The listing builds one solid part. Answer for the finished solid, in the listing's coordinates (mm). Coordinates: 2 decimals unless noted, no trailing zeros. Write each loop counter-clockwise with the first axis right and the second up, starting at its lowest first coordinate (ties: lowest second). Pieces come first, ordered by that corner, then holes. Notation, with made-up numbers: M 39.5,28.25 L 63.5,28.25 A13 cw 63.5,52.25 Z; hole C 46.25,17 d1. An arc over 180 degrees is marked long. Answer as a JSON object with one key per item and string values. Group by question number.
from build123d import *

# Parameters (mm, degrees)
F0_R     = 100
F0_R_2   = 20
F1_DEPTH = 12.5


with BuildPart() as f1:
    # F0 (on Top) → F1 (new body)
    with BuildSketch(Plane.XY):
        with BuildLine():
            ThreePointArc((205.158335, -0.516176), (96.574996, 55.7576), (102.132146, 177.930417))
            ThreePointArc((102.132146, 177.930417), (0, 375), (-102.132146, 177.930417))
            ThreePointArc((-102.132146, 177.930417), (-96.574996, 55.7576), (-205.158335, -0.516176))
            ThreePointArc((-205.158335, -0.516176), (-324.759526, -187.5), (-103.026189, -177.414242))
            ThreePointArc((-103.026189, -177.414242), (0, -111.5152), (103.026189, -177.414242))
            ThreePointArc((103.026189, -177.414242), (324.759526, -187.5), (205.158335, -0.516176))
        make_face()
        Circle(F0_R, mode=Mode.SUBTRACT)
        Circle(F0_R)
        Circle(F0_R_2, mode=Mode.SUBTRACT)
    extrude(amount=F1_DEPTH)


solid = f1.part
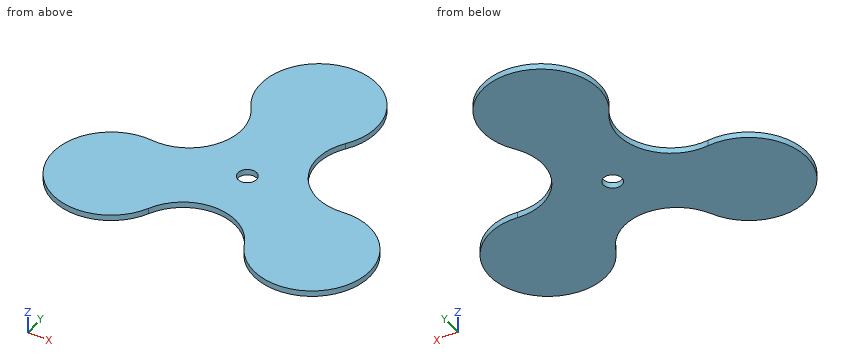
Item 1: A cutting plane is placed at A-A, the plane x = 0. Write down the section's boundary in (y, z).
Item 2: A cutting plane is placed at D-D, the plane x = -144. Write down the section's boundary in (y, z), and give its area (3 significant figures).
Item 3: A cutting plane is placed at C-C, the plane z = 8.5. Write down the section's boundary in (x, y).
Item 4: A flat-ended cylindrical pin translates along its axis: pin 1 Ø5 at (x, z) = (176, 11) entering from -Y. Find the tip coordinate at first contact, or state that the pin passes through.
Item 5: Consider L1, parallel to X at y = -210, z = 8.75; L2, parallel to X at y = -198.5, z = 1; L3, parallel to X at y = 197, z = 11.5. Determine where each line is inside the solid, lowest interval first. Write a range as from..to.
Item 6: A cutting plane is placed at B-B, the plane y = -125. Write down the section's boundary in (x, z).
Answer:
{
 "1": {"outline": "M -111.52,0 L -20,0 L -20,12.5 L -111.52,12.5 Z; M 20,0 L 375,0 L 375,12.5 L 20,12.5 Z"},
 "2": {"outline": "M -226.82,0 L 11.05,0 L 11.05,12.5 L -226.82,12.5 Z", "area": "2,970 mm2"},
 "3": {"outline": "M -205.16,-0.52 A125 ccw long -103.03,-177.41 A113.48 cw 103.03,-177.41 A125 ccw long 205.16,-0.52 A113.48 cw 102.13,177.93 A125 ccw long -102.13,177.93 A113.48 cw Z; hole C 0,0 d40"},
 "4": {"pin 1": "y = -244.08"},
 "5": {"L1": "-308.16..-124.85, 124.85..308.16", "L2": "-317.61..-115.4, 115.4..317.61", "L3": "-113.21..113.21"},
 "6": {"outline": "M -341.51,0 L -53.65,0 L -53.65,12.5 L -341.51,12.5 Z; M 53.65,0 L 341.51,0 L 341.51,12.5 L 53.65,12.5 Z"}
}
